Can you work these out from the model? Positions are in its coordinate system, mm. Face numbers are marked on the shaded views. A direction names the side the tool comes from. Coordinates: 2 decimals unless noted, no trailing zeros. Loops run counter-clockwise (first coordinate to the right, second up) from the corner with the lowest first, then second, coordinate; pieces in that order, holes last.
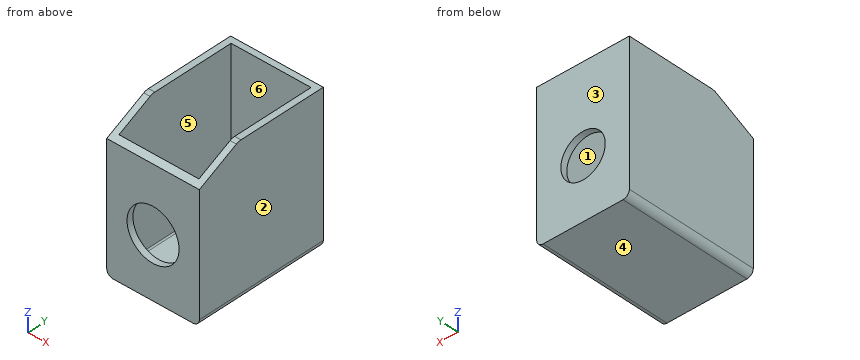
```python
from build123d import *

# Parameters (mm, degrees)
MAINBODYS_W          = 14.6
MAINBODYS_H          = 23
MAIN_BODY_DEPTH      = 10.5
MB_FILLET_R          = 1
SHELL_START          = -6.3
SHELL_MB_OUTLINE_W   = 19
SHELL_MB_OUTLINE_H   = 22
SHELL_MB_DEPTH       = 12.6
TOP_BORE_REACH       = 27.031
TOPBORES_R           = 3.5
BOTTOMBORES_R        = 4.1
BOTTOM_BORE_DEPTH    = 25.197933796
ANGLEDCUT_DEPTH      = 18.19854645
ANGLEDCUT_DEPTH_BACK = 18.19854645
MB_INNER_FILLET_R    = 0.2
AC_F_R               = 1.76


# Read off the part's stored shape, not the designer's step: SHELL MB
with BuildPart() as part:
    # MainBodyS → MAIN BODY (new, symmetric)
    with BuildSketch(Plane(origin=(0, 0, 0), x_dir=(1, 0, 0), z_dir=(0, 1, 0))):
        Rectangle(MAINBODYS_W, MAINBODYS_H)
    extrude(amount=MAIN_BODY_DEPTH, both=True)

    # MB FILLET
    mb_fillet_edges = [part.edges().sort_by_distance(p)[0] for p in [
        (-7.3, 0, -11.5),
        (7.3, 0, -11.5),
    ]]
    fillet(mb_fillet_edges, radius=MB_FILLET_R)

    # SHELL MB outline → SHELL MB (cut)
    with BuildSketch(Plane.YZ.offset(SHELL_START)):
        with Locations((0, 0.5)):
            Rectangle(SHELL_MB_OUTLINE_W, SHELL_MB_OUTLINE_H)
    extrude(amount=SHELL_MB_DEPTH, mode=Mode.SUBTRACT)

    # TopBoreS → TOP BORE (cut, up to next)
    with BuildSketch(Plane(origin=(0, 10.5, 0), x_dir=(1, 0, 0), z_dir=(0, 1, 0)), mode=Mode.PRIVATE) as top_bore_sk1:
        with Locations(Location((0, 2, 0), (0, 0, 270))):
            Circle(TOPBORES_R)
    top_bore_tool1 = extrude(top_bore_sk1.sketch, amount=-TOP_BORE_REACH, mode=Mode.PRIVATE) & part.part
    add(top_bore_tool1.solids().sort_by_distance((0, 10.5, -2))[0], mode=Mode.SUBTRACT)

    # BottomBoreS → BOTTOM BORE (cut, through all)
    with BuildSketch(Plane(origin=(0, -9.5, 0), x_dir=(1, 0, 0), z_dir=(0, 1, 0))):
        with Locations(Location((0, 2, 0), (0, 0, 270))):
            Circle(BOTTOMBORES_R)
    extrude(amount=-BOTTOM_BORE_DEPTH, mode=Mode.SUBTRACT)

    # AngledCutS → AngledCut (cut, two sides: drawn at the far end of the back side and taken through both)
    with BuildSketch(Plane(origin=(0, 0, 0), x_dir=(0, 0, -1), z_dir=(1, 0, 0)).offset(-ANGLEDCUT_DEPTH_BACK)):
        Polygon((-41.74417665, 56.547529947), (-11.5, -3.85), (-8.17, -10.5), (22.07417665, -70.897529947), (-98.720883244, -131.385883248), (-162.539236545, -3.940823353), align=None)
    extrude(amount=ANGLEDCUT_DEPTH + ANGLEDCUT_DEPTH_BACK, mode=Mode.SUBTRACT)

    # MB INNER FILLET
    mb_inner_fillet_edges = [part.edges().sort_by_distance(p)[0] for p in [
        (6.3, 0, -10.5),
        (-6.3, 0, -10.5),
    ]]
    fillet(mb_inner_fillet_edges, radius=MB_INNER_FILLET_R)

    # AC F
    ac_f_edges = [part.edges().sort_by_distance(p)[0] for p in [
        (-6.8, -3.85, 11.5),
        (6.8, -3.85, 11.5),
    ]]
    fillet(ac_f_edges, radius=AC_F_R)


solid = part.part
```
Item 1: I need wall thicknesses on line 1 along Y through (x, z) = (-5.5, -9.25); line 2 along X through (y, z) = (4.25, -5.25); line 3 along X through (y, z) = (-9.95, -2). Which ranges of each line are inside material? Lowest first, please.
Results are:
line 1: y = -10.5 to -9.5, 9.5 to 10.5
line 2: x = -7.3 to -6.3, 6.3 to 7.3
line 3: x = -7.3 to -4.1, 4.1 to 7.3
Item 2: I'm going to push a flat-ended pin straight in: P1, Ø4, axis at x = 1, y = -0.5, coming from the +Z side. Where does the tip first touch, or does it pass through?
Results are:
P1: stops at z = -10.5
Item 3: Suppose I cut it at B-B, the plane z = 7. Please give me the cut outline in (x, y), plus the area to 3 significant figures.
Results are:
outline: (-7.3, -10.5) - (7.3, -10.5) - (7.3, 10.5) - (-7.3, 10.5) - close; hole (-6.3, -9.5) - (6.3, -9.5) - (6.3, 9.5) - (-6.3, 9.5) - close
area: 67.2 mm2
Item 4: On a 3-axis mill with a long thin cutter (end or side, diameter ignored), from which of +Z, -Z, +X, -X, +Y, -Y can I reach the whole of each face in a straight line? I mean the marked faces 1 and 2. Say none if no direction works.
Results are:
face 1: +Z
face 2: +Z, -Z, +X, +Y, -Y
Item 5: Suppose I cut it at A-A, the plane x = 0. Please give me the cut outline in (y, z), plus the area to 3 significant figures.
Results are:
outline: (-10.5, -11.5) - (10.5, -11.5) - (10.5, -5.5) - (9.5, -5.5) - (9.5, -10.5) - (-9.5, -10.5) - (-9.5, -6.1) - (-10.5, -6.1) - close; (-10.5, 2.1) - (-9.5, 2.1) - (-9.5, 8.67) - (-10.5, 8.17) - close; (9.5, 1.5) - (10.5, 1.5) - (10.5, 11.5) - (9.5, 11.5) - close
area: 46.7 mm2
Item 6: Suppose I cut it at C-C, the plane y = 7.5. Please give me the cut outline in (x, z), plus the area to 3 significant figures.
Results are:
outline: (-7.3, -10.5) arc R1 ccw to (-6.3, -11.5) - (6.3, -11.5) arc R1 ccw to (7.3, -10.5) - (7.3, 11.5) - (6.3, 11.5) - (6.3, -10.3) arc R0.2 cw to (6.1, -10.5) - (-6.1, -10.5) arc R0.2 cw to (-6.3, -10.3) - (-6.3, 11.5) - (-7.3, 11.5) - close
area: 58.2 mm2
Item 7: We'd pull the mould along Y, two halves only. Please class the marked faces 3, 4, 5 and 6: +Y half, -Y half, draft (parallel to the pull), parting line (faces both ways), or undercut.
Results are:
face 3: +Y half
face 4: draft
face 5: undercut
face 6: undercut
Item 8: Suppose I cut it at D-D, the plane z = -2. Please give me the cut outline in (x, y), plus the area to 3 significant figures.
Results are:
outline: (-7.3, -10.5) - (-4.1, -10.5) - (-4.1, -9.5) - (-6.3, -9.5) - (-6.3, 9.5) - (-3.5, 9.5) - (-3.5, 10.5) - (-7.3, 10.5) - close; (3.5, 9.5) - (6.3, 9.5) - (6.3, -9.5) - (4.1, -9.5) - (4.1, -10.5) - (7.3, -10.5) - (7.3, 10.5) - (3.5, 10.5) - close
area: 52.0 mm2
